Autodesk Inventor part; units mm, degrees
ref_plane "ip_st_1_XY" through (0, 0, 0) normal (1, 0, 0) x (0, 0, -1)
ref_plane "ip_st_1_YZ" through (0, 0, 0) normal (0, 0, -1) x (0, 1, 0)
ref_plane "ip_st_1_ZX" through (0, 0, 0) normal (0, 1, 0) x (1, 0, 0)
sketch "Sketch_1" plane through (0, 0, 0) normal (0, 0, 1) x (1, 0, 0)
  line L0 (3, 0) -> (0, 0)
  line L1 (0, 4.655) -> (0.1875, 4.655)
  line L2 (0.1875, 4.655) -> (0.1875, 4.375)
  line L3 (0.1875, 4.375) -> (1.0316, 4.375)
  arc A0 (1.9684, 4.375) -> (1.0316, 4.375) centre (1.5, 4) ccw
  line L4 (1.9684, 4.375) -> (2.8125, 4.375)
  line L5 (2.8125, 4.375) -> (2.8125, 4.655)
  line L6 (2.8125, 4.655) -> (3, 4.655)
  line L7 (3, 4.655) -> (3, 5.5)
  arc A1 (3, 5.5) -> (2.9, 5.6) centre (2.9, 5.5) ccw
  line L8 (2.9, 5.6) -> (2.4, 5.6)
  line L9 (2.4, 5.6) -> (2.4, 5)
  line L10 (2.4, 5) -> (0.1, 5)
  arc A2 (0.1, 5) -> (0, 4.9) centre (0.1, 4.9) ccw
  line L11 (0, 4.9) -> (0, 4.655)
revolve "Revolution1" add sketch "Sketch_1" angle 360 about axis through (3, 0, 0) along (1, 0, 0)
ref_plane "ip_st_1_XY" through (0, 0, 0) normal (1, 0, 0) x (0, 0, -1)
ref_plane "ip_st_1_YZ" through (0, 0, 0) normal (0, 0, -1) x (0, 1, 0)
ref_plane "ip_st_1_ZX" through (0, 0, 0) normal (0, 1, 0) x (1, 0, 0)
ref_plane "ip_st_2_XY" through (2.8125, 0, 0) normal (-1, 0, 0) x (0, 0, -1)
ref_plane "ip_st_2_YZ" through (2.8125, 0, 0) normal (0, 0, -1) x (0, -1, 0)
ref_plane "ip_st_2_ZX" through (2.8125, 0, 0) normal (0, -1, 0) x (-1, 0, 0)
properties part number "MF106ZZ1 Outer Ring"
Here's how the part is built. I have some questions about the finished solid (model axes, mm). A direction names the side the tool comes from. Coordinates: 2 decimals unless noted, no trailing zeros. Order: outer loops, then holes, each group sorted by start corner. A loop starts at its lowest first (then second) coordinate and runs counter-clockwise, first axis right, second up.
Item 1: If we mould it in two halves opening along Y, with no side actions, what happens to faces 3 (the face through (2.396, -3.472, -2.662)), 4 (the face through (0.615, -3.472, -2.662)), 5 (the face through (2.4, -2, 5)), 6 (the face through (2.646, -5.595, -0.246))? For each: +Y half, -Y half, draft (parallel to the pull), parting line (faces both ways), or undercut.
Result sheet:
face 3: undercut
face 4: undercut
face 5: draft
face 6: parting line
Item 2: If we section it at D-D on x = 2.65: List the corners of the cut face in (y, z) for me (3 decimals), plus the area to 3 significant figures.
Result sheet:
outline: circle Ø11.2 at (0, 0); hole circle Ø8.75 at (0, 0)
area: 38.4 mm2
Item 3: If we section it at C-C on x = 1.5: List the corners of the cut face in (y, z) for me, plus the area to 3 significant figures.
Result sheet:
outline: circle Ø10 at (0, 0); hole circle Ø9.2 at (0, 0)
area: 12.1 mm2
Item 4: For faces 1 (the face through (3, -5, 1)), 2 (the face through (1.23, -1.08, 4.88)), which set-ups out of +Z, -Z, +X, -X, +Y, -Y let a thin tool reach every point of the face, with its end or its side?
Result sheet:
face 1: +Z, -Z, +X, +Y, -Y
face 2: -X
Item 5: I need wall thicknesses on line 1 (Z direction, x = 2.25, y = 0) (3 decimals); line 2 (Z direction, x = 2.9, y = 0) (3 decimals); line 3 (X direction, y = 2, z = 4). Which ranges of each line are inside material? Lowest first, please.
Result sheet:
line 1: z = -5 to -4.375, 4.375 to 5
line 2: z = -5.6 to -4.655, 4.655 to 5.6
line 3: x = 0.19 to 1.13, 1.87 to 2.81
